from build123d import *

# Parameters (mm, degrees)
EXTRUDE_1_DEPTH      = 30
SKETCH_2_W           = 20
SKETCH_2_H           = 10.454482672
CUT_EXTRUDE_1_DEPTH  = 52.134626233
CUT_EXTRUDE_4_DEPTH  = 52.134626233
SKETCH_4_R           = 4
SKETCH_4_R_2         = 2
EXTRUDE_2_DEPTH      = 30
CUT_EXTRUDE_5_DEPTH  = 53.403183519
SKETCH_6_R           = 4
SKETCH_6_R_2         = 2
EXTRUDE_3_DEPTH      = 30
CUT_EXTRUDE_START    = -10
SKETCH_7_R           = 4
SKETCH_7_R_2         = 2
CUT_EXTRUDE_8_DEPTH  = 10
SKETCH_8_R           = 4
SKETCH_8_R_2         = 2
CUT_EXTRUDE_9_DEPTH  = 10
CUT_EXTRUDE_START_2  = -20
SKETCH_9_R           = 4
SKETCH_9_R_2         = 2
CUT_EXTRUDE_10_DEPTH = 10
EXTRUDE_4_DEPTH      = 30
SKETCH_12_W          = 33.381197846
SKETCH_12_H          = 2
EXTRUDE_5_DEPTH      = 30
EXTRUDE_6_DEPTH      = 30
SKETCH_13_W          = 20
SKETCH_13_H          = 3.5
CUT_EXTRUDE_11_DEPTH = 30


with BuildPart() as part:
    # 스케치1 → 보스-돌출1 (new body)
    with BuildSketch(Plane(origin=(0, 0, 0), x_dir=(0, 0, -1), z_dir=(1, 0, 0))):
        Polygon((0, 0), (9.5, 16.454482672), (28.5, 16.454482672), (38, 0), align=None)
    extrude(amount=EXTRUDE_1_DEPTH)

    # 스케치2 → 컷-돌출1 (cut, through all)
    with BuildSketch(Plane.XY):
        with Locations((15, 8.227241336)):
            Rectangle(SKETCH_2_W, SKETCH_2_H)
    extrude(amount=-CUT_EXTRUDE_1_DEPTH, mode=Mode.SUBTRACT)

    # 스케치3 → 컷-돌출4 (cut, through all)
    with BuildSketch(Plane(origin=(30, 0, 0), x_dir=(0, 0, -1), z_dir=(1, 0, 0))):
        with BuildLine():
            Line((33.690598923, 7.464101615), (37.690598923, 0.535898385))
            ThreePointArc((37.690598923, 0.535898385), (39.154700538, 2), (39.690598923, 4))
            ThreePointArc((39.690598923, 4), (37.690598923, 7.464101615), (33.690598923, 7.464101615))
        make_face()
        with BuildLine():
            ThreePointArc((35.690598923, 0), (36.725875104, 0.136296695), (37.690598923, 0.535898385))
            Line((37.690598923, 0.535898385), (33.690598923, 7.464101615))
            ThreePointArc((33.690598923, 7.464101615), (31.826895618, 2.96472382), (35.690598923, 0))
        make_face()
        with BuildLine():
            Line((35.690598923, 0), (38, 0))
            Line((38, 0), (37.690598923, 0.535898385))
            ThreePointArc((37.690598923, 0.535898385), (36.725875104, 0.136296695), (35.690598923, 0))
        make_face()
    extrude(amount=-CUT_EXTRUDE_4_DEPTH, mode=Mode.SUBTRACT)

    # 스케치4 → 보스-돌출2 (add)
    with BuildSketch(Plane(origin=(30, 0, 0), x_dir=(0, 0, -1), z_dir=(1, 0, 0))):
        with Locations((35.690598923, 4)):
            Circle(SKETCH_4_R)
        with Locations((35.690598923, 4)):
            Circle(SKETCH_4_R_2, mode=Mode.SUBTRACT)
    extrude(amount=-EXTRUDE_2_DEPTH)

    # 스케치5 → 컷-돌출5 (cut, through all)
    with BuildSketch(Plane(origin=(30, 0, 0), x_dir=(0, 0, -1), z_dir=(1, 0, 0))):
        with BuildLine():
            Line((4.309401077, 7.464101615), (0.309401077, 0.535898385))
            ThreePointArc((0.309401077, 0.535898385), (1.274124896, 0.136296695), (2.309401077, 0))
            ThreePointArc((2.309401077, 0), (5.137828202, 1.171572875), (6.309401077, 4))
            ThreePointArc((6.309401077, 4), (5.773502692, 6), (4.309401077, 7.464101615))
        make_face()
        with BuildLine():
            ThreePointArc((4.309401077, 7.464101615), (-1.154700538, 6), (0.309401077, 0.535898385))
            Line((0.309401077, 0.535898385), (4.309401077, 7.464101615))
        make_face()
        with BuildLine():
            ThreePointArc((2.309401077, 0), (1.274124896, 0.136296695), (0.309401077, 0.535898385))
            Line((0.309401077, 0.535898385), (0, 0))
            Line((0, 0), (2.309401077, 0))
        make_face()
    extrude(amount=-CUT_EXTRUDE_5_DEPTH, mode=Mode.SUBTRACT)

    # 스케치6 → 보스-돌출3 (add)
    with BuildSketch(Plane(origin=(30, 0, 0), x_dir=(0, 0, -1), z_dir=(1, 0, 0))):
        with Locations((2.309401077, 4)):
            Circle(SKETCH_6_R)
        with Locations((2.309401077, 4)):
            Circle(SKETCH_6_R_2, mode=Mode.SUBTRACT)
    extrude(amount=-EXTRUDE_3_DEPTH)

    # 스케치7 → 컷-돌출8 (cut)
    with BuildSketch(Plane(origin=(30, 0, 0), x_dir=(0, 0, -1), z_dir=(1, 0, 0)).offset(CUT_EXTRUDE_START)):
        with Locations((2.309401077, 4)):
            Circle(SKETCH_7_R)
        with Locations((2.309401077, 4)):
            Circle(SKETCH_7_R_2, mode=Mode.SUBTRACT)
    extrude(amount=-CUT_EXTRUDE_8_DEPTH, mode=Mode.SUBTRACT)

    # 스케치8 → 컷-돌출9 (cut)
    with BuildSketch(Plane(origin=(30, 0, 0), x_dir=(0, 0, -1), z_dir=(1, 0, 0))):
        with Locations((35.690598923, 4)):
            Circle(SKETCH_8_R)
        with Locations((35.690598923, 4)):
            Circle(SKETCH_8_R_2, mode=Mode.SUBTRACT)
    extrude(amount=-CUT_EXTRUDE_9_DEPTH, mode=Mode.SUBTRACT)

    # 스케치9 → 컷-돌출10 (cut)
    with BuildSketch(Plane(origin=(30, 0, 0), x_dir=(0, 0, -1), z_dir=(1, 0, 0)).offset(CUT_EXTRUDE_START_2)):
        with Locations((35.690598923, 4)):
            Circle(SKETCH_9_R)
        with Locations((35.690598923, 4)):
            Circle(SKETCH_9_R_2, mode=Mode.SUBTRACT)
    extrude(amount=-CUT_EXTRUDE_10_DEPTH, mode=Mode.SUBTRACT)

    # 스케치11 → 보스-돌출4 (add)
    with BuildSketch(Plane(origin=(30, 0, 0), x_dir=(0, 0, -1), z_dir=(1, 0, 0))):
        with BuildLine():
            Line((4.309401077, 7.464101615), (33.690598923, 7.464101615))
            ThreePointArc((33.690598923, 7.464101615), (31.826895618, 2.96472382), (35.690598923, 0))
            Line((35.690598923, 0), (2.309401077, 0))
            ThreePointArc((2.309401077, 0), (6.173104382, 2.96472382), (4.309401077, 7.464101615))
        make_face()
    extrude(amount=-EXTRUDE_4_DEPTH)

    # 스케치12 → 보스-돌출5 (add)
    with BuildSketch(Plane.ZY):
        with Locations((-19, -1)):
            Rectangle(SKETCH_12_W, SKETCH_12_H)
    extrude(amount=-EXTRUDE_5_DEPTH)

    # 스케치14 → 보스-돌출6 (add)
    with BuildSketch(Plane(origin=(30, 0, 0), x_dir=(0, 0, -1), z_dir=(1, 0, 0))):
        Polygon((28.5, 16.454482672), (26.767949192, 19.454482672), (11.232050808, 19.454482672), (9.5, 16.454482672), align=None)
    extrude(amount=-EXTRUDE_6_DEPTH)

    # 스케치13 → 컷-돌출11 (cut)
    with BuildSketch(Plane(origin=(0, 0, -35.690598923), x_dir=(-1, 0, 0), z_dir=(0, 0, -1))):
        with Locations((-15, 15.204482672)):
            Rectangle(SKETCH_13_W, SKETCH_13_H)
    extrude(amount=-CUT_EXTRUDE_11_DEPTH, mode=Mode.SUBTRACT)


solid = part.part
Source: CAD feature listing. Evaluate the final solid. Frame: model axes, mm. A direction names the side the tool comes from. Coordinates: 2 decimals unless noted, no trailing zeros. Loops run counter-clockwise (first coordinate to the right, second up) from the corner with the lowest first, then second, coordinate; pieces in that order, holes last. Notation, with made-up numbers: (35.5, 69) - (51.5, 69) arc R6 ccw to (51.5, 80) - close; hole circle Ø1 at (86.25, -22.75). An arc over 180 degrees is marked (long way). One line per item, written item: value. Start each with the question number.
1. Section A-A (x = 15.75). Return the cut outline in (y, z).
2. Section B-B (y = 4). Return the cut outline in (x, z), and give its area (3 significant figures).
3. Set-up query: faces 1 (the flat face through (15, -1, -2.309)), 2 (the flat face through (15, -1, -35.691)). Return all of +Z, -Z, +X, -X, +Y, -Y with unobstructed straight access to the full face (end or side cutting, diameter ignored); none if empty.
4. Ray query, L1, parallel to X at y = 11.5, z = -21; L2, parallel to Y at x = 24.25, z = -16.5; L3, parallel to X at y = 1, z = -4. Return the intervals inside material, ascending.
5. Section C-C (z = -12). Return the cut outline in (x, y).
6. Mould query, pull axis X, two halves, no side actions, for faces 3 (the flat face through (15, 7.464, -19)), 4 (the flat face through (15, 16.954, -19)), 5 (the flat face through (20, 6, -37)), 6 (the cylindrical face through (5.07, 3.036, -31.809)). Classes: pulls with the +X half, pulls with the -X half, needs draft (parallel to the pull), parting line crosses it, or undercut.
7. Section D-D (x = 27.5). Return the cut outline in (y, z).
8. Contact query for flat-ended pins moving along their axis: P1, Ø6, axis at y = 13, z = -10, coming from the -X side; P2, Ø4, axis at x = 20.5, y = 16, coming from the -Z side; P3, Ø3, axis at x = 27, y = 0.5, coming from the +Z side; P4, Ø4, axis at x = 5.5, y = 10, coming from the -Z side. Output: stop coordinate, or through.
Verdict:
1. outline: (-2, -35.69) - (0, -35.69) arc R4 ccw (long way) to (7.46, -33.69) - (7.46, -4.31) arc R4 cw to (0, -2.31) - (-2, -2.31) - close; (16.95, -28.21) - (19.45, -26.77) - (19.45, -11.23) - (16.95, -9.79) - close; hole circle Ø4 at (4, -35.69)
2. outline: (0, -31.69) - (10, -31.69) - (10, -33.69) - (20, -33.69) - (20, -31.69) - (30, -31.69) - (30, -4.31) - (20, -4.31) - (20, -6.31) - (10, -6.31) - (10, -4.31) - (0, -4.31) - close; (0, -0.31) - (10, -0.31) - (10, 1.69) - (0, 1.69) - close; (10, -39.69) - (20, -39.69) - (20, -37.69) - (10, -37.69) - close; (20, -0.31) - (30, -0.31) - (30, 1.69) - (20, 1.69) - close
2. area: 881 mm2
3. face 1: +Z, +X, -X, -Y
3. face 2: -Z, +X, -X, -Y
4. L1: x = 0 to 5, 25 to 30
4. L2: y = -2 to 7.46, 16.95 to 19.45
4. L3: x = 0 to 10, 20 to 30
5. outline: (0, -2) - (30, -2) - (30, 19.45) - (0, 19.45) - close; hole (5, 7.46) - (25, 7.46) - (25, 16.95) - (5, 16.95) - close
6. face 3: undercut
6. face 4: undercut
6. face 5: pulls with the +X half
6. face 6: needs draft
7. outline: (-2, -35.69) - (0, -35.69) arc R4 cw to (7.46, -33.69) - (19.45, -26.77) - (19.45, -11.23) - (7.46, -4.31) arc R4 ccw (long way) to (0, -2.31) - (-2, -2.31) - close; hole circle Ø4 at (4, -2.31)
8. P1: stops at x = 0
8. P2: stops at z = -28.21
8. P3: stops at z = 1.15
8. P4: stops at z = -33.34
